from build123d import *

# Parameters (mm, degrees)
F0_W     = 111.1538112164
F0_H     = 49.8025715351
F1_DEPTH = 50.8
F2_R     = 5.08
F3_SIZE  = 25.4
F4_W     = 25.4
F4_H     = 49.8025715351
F5_DEPTH = 19.05
F6_R     = 8.0573195259
F7_F1_R  = 5.08
F7_F2_R  = 5.08
F7_F3_R  = 5.08
F7_F4_R  = 5.08


# Not quite as in the source:
# - a feature of the source that left no trace in its solid (it failed there, or was rolled back) is left out


with BuildPart() as f1:
    # F0 (on Front) → F1 (new body)
    with BuildSketch(Plane.XZ):
        Rectangle(F0_W, F0_H)
    extrude(amount=F1_DEPTH)

    # F2
    f2_edges = [f1.edges().sort_by_distance(p)[0] for p in [
        (-55.576906, -50.8, 0),
    ]]
    fillet(f2_edges, radius=F2_R)

    # F3
    f3_edges = [f1.edges().sort_by_distance(p)[0] for p in [
        (55.576906, -50.8, 0),
    ]]
    chamfer(f3_edges, length=F3_SIZE)

    # F4 (on face) → F5 (join)
    with BuildSketch(Plane.YZ.offset(55.5769056082)):
        with Locations((-12.7, 0)):
            Rectangle(F4_W, F4_H)
    extrude(amount=F5_DEPTH)

    # F6
    f6_edges = [f1.edges().sort_by_distance(p)[0] for p in [
        (74.626906, -25.4, 0),
    ]]
    fillet(f6_edges, radius=F6_R)

    # F7: fillet of radius 5.08 on 4 edges, made by hand

    # F7_f1
    f7_f1_edges = [f1.edges().sort_by_distance(p)[0] for p in [
        (55.5769056082, -25.4, 0),
    ]]
    fillet(f7_f1_edges, radius=F7_F1_R)

    # F7_f2
    f7_f2_edges = [f1.edges().sort_by_distance(p)[0] for p in [
        (30.1769056082, -50.8, 0),
    ]]
    fillet(f7_f2_edges, radius=F7_F2_R)

    # F7_f3
    f7_f3_edges = [f1.edges().sort_by_distance(p)[0] for p in [
        (42.8769056082, -38.1, 24.9012857676),
    ]]
    fillet(f7_f3_edges, radius=F7_F3_R)

    # F7_f4
    f7_f4_edges = [f1.edges().sort_by_distance(p)[0] for p in [
        (42.8769056082, -38.1, -24.9012857676),
    ]]
    fillet(f7_f4_edges, radius=F7_F4_R)


solid = f1.part
Geometry: final body of the model. Coordinates: model frame, mm. A direction names the side the tool comes from. Give positions to 0.01 mm unless a question says otherwise; leave off trailing zeros. Write each loop counter-clockwise with the first axis right and the second up, starting at its lowest first coordinate (ties: lowest second). Pieces come first, ordered by that corner, then holes. Notation, with made-up numbers: M 32.5,66.25 L 56.5,66.25 A30 ccw 56.5,103.25 Z; hole C 73.25,15 d4. An arc over 180 degrees is marked long. Answer in a Markdown table with one row per item. Add a question column.
(1) First-contact query: pin 1 (10 mm diameter, centred on x = 61.5, z = 0, fed in from -Y); pin 2 (4 mm diameter, centred on x = 52.5, y = -30.5, fed in from +Z); pin 3 (6 mm diameter, centred on x = 42.5, z = 18.5, fed in from -Y). Flat tips, straight axial feed; report the tip coordinate or a pass-through.
(2) Reachability of faces 1 (the cylindrical face through (62.188, -23.951, 23.374)), 2 (the cylindrical face through (62.188, -23.951, -23.374)), 3 (the cylindrical face through (-54.1, -23.2, -23.4)) from +Z, -Z, +X, -X, +Y, -Y: full face, straight path, thin tool, end or side. Return the list, or none.
(3) Section A-A on z = 16. Return loops of the section in (x, y), and give its area (3 significant figures).
(4) Ray query, line 1 (Z direction, x = 48, y = -26.5); line 2 (X direction, y = -17.5, z = 16); line 3 (X direction, y = -30.5, z = 17.5). Return the intervals inside material, ascending.
Result set:
| question | item | result |
|---|---|---|
| 1 | pin 1 | stops at y = -25.54 |
| 1 | pin 2 | stops at z = 22.16 |
| 1 | pin 3 | stops at y = -41.48 |
| 2 | face 1 | +Z, +X, -Y |
| 2 | face 2 | -Z, +X, -Y |
| 2 | face 3 | -Z, -X, +Y, -Y |
| 3 | outline | M -55.58,-45.72 A5.08 ccw -50.5,-50.8 L 28.07,-50.8 A5.08 ccw 31.66,-49.31 L 54.09,-26.89 A5.08 cw 57.68,-25.4 L 66.57,-25.4 A8.06 ccw 74.63,-17.34 L 74.63,0 L -55.58,0 Z |
| 3 | area | 5,790 mm^2 |
| 4 | line 1 | z = -24.88 to 24.88 |
| 4 | line 2 | x = -55.58 to 74.63 |
| 4 | line 3 | x = -55.58 to 50.48 |
